CAD build for the part. Positions are in the model's coordinates, mm. Face numbers are marked on the shaded views. Coordinates: 2 decimals unless noted, no trailing zeros. Write each loop counter-clockwise with the first axis right and the second up, starting at its lowest first coordinate (ties: lowest second). Pieces come first, ordered by that corner, then holes. Notation, with made-up numbers: M 82.25,88 L 91.25,88 A13 ccw 91.25,99 Z; hole C -8,39 d6. An arc over 180 degrees is marked long. Put each result on its own line as item: value. Start each with the question number.
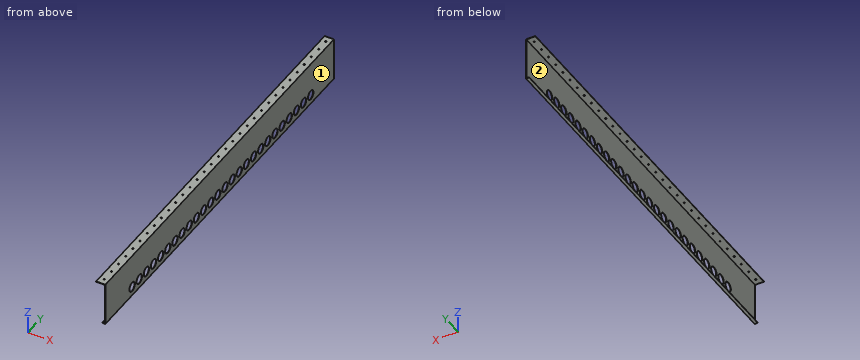
Autodesk Inventor part; units mm, degrees
ref_plane "YZ Plane" through (0, 0, 0) normal (1, 0, 0) x (0, 1, 0)
ref_plane "XZ Plane" through (0, 0, 0) normal (0, 1, 0) x (-1, 0, 0)
ref_plane "XY Plane" through (0, 0, 0) normal (0, 0, 1) x (1, 0, 0)
sketch "Sketch1" plane through (0, 0, 0) normal (0, 1, 0) x (-1, 0, 0)
  line L0 (0, 0) -> (0, 88.9)
  line L1 (0, 88.9) -> (19.05, 88.9)
  line L2 (19.05, 88.9) -> (19.05, 88.265)
  line L3 (19.05, 88.265) -> (0.635, 88.265)
  line L4 (0.635, 88.265) -> (0.635, 0.635)
  line L5 (0, 0) -> (6.35, 0)
  line L6 (6.35, 0) -> (6.35, 0.635)
  line L7 (6.35, 0.635) -> (0.635, 0.635)
  dimension "d0" = 88.9
  dimension "d1" = 19.05
  dimension "d2" = 0.635
  dimension "d4" = 0.635
  dimension "d7" = 6.35
extrude "Extrusion1" add sketch "Sketch1" along normal blind 812.8
sketch "Sketch2" plane through (-19.05, 0, 88.9) normal (0, 0, 1) x (1, 0, 0)
  line L0 (19.05, 0) -> (0, 0)
  line L1 (19.05, 0) -> (19.05, 812.8)
  line L2 (9.525, 0) -> (9.525, 12.7)
  line L3 (0, 0) -> (0, 812.8)
  line L4 (9.525, 12.7) -> (9.525, 27.5524) construction
  dimension "d8" = 12.7
hole "Hole1" at (-9.525, 12.7, 88.9) direction (0, 0, -1) diameter 2.54 end through all
pattern_linear "Rectangular Pattern1" count 32 spacing 25.4 along (0, 1, 0) of "Hole1"
sketch "Sketch3" plane through (0, 0, 88.9) normal (1, 0, 0) x (0, 0, -1)
  line L0 (88.9, 0) -> (0, 0)
  line L1 (88.9, 0) -> (88.9, 812.8)
  line L2 (0, 0) -> (0, 812.8)
  line L3 (69.85, 0) -> (69.85, 95.25)
  line L4 (69.85, 95.25) -> (69.85, 151.65) construction
  dimension "d19" = 19.05
  dimension "d20" = 95.25
hole "Hole2" at (0, 95.25, 19.05) direction (-1, 0, 0) diameter 19.05 end through all
pattern_linear "Rectangular Pattern2" count 26 spacing 25.4 along (0, 1, 0) of "Hole2"
equation "\"d14\" = Thickness"
equation "\"d26\" = Thickness"
equation "\"BendRadius\" = Thickness"
equation "\"BendReliefWidth\" = Thickness"
equation "\"BendReliefDepth\" = 0.5 * Thickness"
equation "\"CornerReliefSize\" = 4 * Thickness"
equation "\"MinimumRemnant\" = 2 * Thickness"
equation "\"TransitionRadius\" = BendRadius"
equation "\"JacobiRadiusSize\" = BendRadius"
equation "\"GapSize\" = Thickness"
properties part number "2014 Sidings"
(1) Slice it at C-C, the plane z = 63. Write the cut outline in (x, y) (3 decimals).
(2) Slice it at A-A, the plane y = 759. Write the cut outline in (x, z) (3 decimals), then the cut area to 3 significant figures.
(3) Drill centre lines: line 1 (X direction, y = 571.5, z = 88.45) (3 decimals); line 2 (Z direction, x = -0.2, y = 323.85) (3 decimals); line 3 (Z direction, x = -4.25, y = 521.5) (3 decimals). Where is each one in solid material? Low to high. Write a range as [from, to].
(4) Slice it at B-B, the plane x = -15.5. Write the cut outline in (y, z) (3 decimals), then the cut area to 3 significant figures.
(5) Drop flat-ended pins along their axis: pin 1 (4 mm diameter, centred on x = -9.525, y = 571.5, fed in from +Z); pin 2 (11.5 mm diameter, centred on y = 425.45, z = 19.05, fed in from -X); pin 3 (22 mm diameter, centred on y = 298.45, z = 19.05, fed in from -X) (3 decimals); pin 4 (4 mm diameter, centred on x = -9.525, y = 114.3, fed in from -Z) (3 decimals). Give the stop position or say it passes through.
(6) Two-plate mould, pull along Z, no slides. Class the marked faces 1 and 2: +Z half, -Z half, draft (parallel to the pull), parting line (faces both ways), or undercut.
Result set:
1. outline: M -0.635,0 L 0,0 L 0,812.8 L -0.635,812.8 Z
2. outline: M -19.05,88.265 L -0.635,88.265 L -0.635,0.635 L -6.35,0.635 L -6.35,0 L 0,0 L 0,88.9 L -19.05,88.9 Z
2. area: 71.8 mm^2
3. line 1: x = [-19.05, -10.795], [-8.255, 0]
3. line 2: z = [0, 9.525], [28.575, 88.9]
3. line 3: z = [0, 0.635], [88.265, 88.9]
4. outline: M 0,88.265 L 812.8,88.265 L 812.8,88.9 L 0,88.9 Z
4. area: 516 mm^2
5. pin 1: stops at z = 88.9
5. pin 2: passes through
5. pin 3: stops at x = -0.635
5. pin 4: stops at z = 88.265
6. face 1: draft
6. face 2: undercut
